Design review of the part built by this model. Coordinates are the model's own, in mm. A direction names the side the tool comes from. Round coordinates to 2 decimals unless told otherwise and drop trailing zeros. Loops run counter-clockwise (first coordinate to the right, second up) from the corner with the lowest first, then second, coordinate; pieces in that order, holes last. Notation, with made-up numbers: (33.5, -40) - (38.5, -40) arc R17 cw to (38.5, -20) - close; hole circle Ø7 at (65, 23.5). An arc over 180 degrees is marked (long way). Return JSON: item names as keys, results as strings. Group by question number.
(1) Wall thickness on L1, parallel to X at y = 4.75, z = 0; L2, parallel to X at y = -10, z = 11.5; L3, parallel to Y at x = 57, z = -0.5: over which ranges is each line inside the solid? List them lowest first. Write a range as [from, to].
(2) For faces 1 (the flat face through (68.58, 0, 0)), 2 (the cylindrical face through (36.403, -7.559, -5.796)), list the 3-axis set-ups (+Z, -Z, +X, -X, +Y, -Y) from which the entire face can be reached by the end or side of a thin tool; tool diameter is ignored.
(3) We need section C-C, the plane x = 24. Write out the cut boundary in (y, z) (3 decimals), and give its area (3 significant figures).
(4) Clearance check with flat-ended pins moving along their axes: pin 1 (10 mm diameter, centred on x = 60.5, z = -10.5, fed in from +Y); pin 2 (8 mm diameter, centred on x = 55, z = 5.5, fed in from -Y); pin 3 (3 mm diameter, centred on x = 16, z = 5, fed in from +Y); pin 4 (4.5 mm diameter, centred on x = 59.95, z = 0, fed in from -Y). State where each tip first meets the part, or that it passes through.
(5) We need section D-D, the plane z = -11.5. Write out the cut boundary in (x, y).
(6) We need section A-A, the plane z = 0. Write out the cut boundary in (x, y) (3 decimals).
(7) The part is to be moulded in two halves that separate along X. For faces 3 (the cylindrical face through (57.566, -0.133, 0.105)), 4 (the flat face through (6.35, 7, -7)), 5 (the cylindrical face through (3.131, -3.441, -15.497)), say which applies: pulls with the +X half, pulls with the -X half, needs draft (parallel to the pull), parting line crosses it, or undercut.
(8) We need section B-B, the plane y = 0. Write out the cut boundary in (x, z) (3 decimals).
from build123d import *

# Parameters (mm, degrees)
F0_R     = 15.875
F1_DEPTH = 6.35
F2_R     = 9.525
F3_DEPTH = 62.23
F4_R     = 1.27
F5_R     = 2.3876
F6_DEPTH = 12.7


with BuildPart() as f1:
    # F0 (on Right) → F1 (new body)
    with BuildSketch(Plane.YZ):
        Circle(F0_R)
    extrude(amount=F1_DEPTH)

    # F2 (on face) → F3 (join)
    with BuildSketch(Plane.YZ.offset(6.35)):
        Circle(F2_R)
    extrude(amount=F3_DEPTH)

    # F4
    f4_edges = [f1.edges().sort_by_distance(p)[0] for p in [
        (68.58, -9.525, 0),
    ]]
    fillet(f4_edges, radius=F4_R)

    # F5 (on Front) → F6 (cut, symmetric)
    with BuildSketch(Plane.XZ):
        with Locations((59.951451, 0)):
            Circle(F5_R)
    extrude(amount=F6_DEPTH, both=True, mode=Mode.SUBTRACT)


solid = f1.part
Solutions:
{
 "1": {"L1": "[0, 57.56], [62.34, 68.58]", "L2": "[0, 6.35]", "L3": "[-9.51, 9.51]"},
 "2": {"face 1": "+Z, -Z, +X, +Y, -Y", "face 2": "+X"},
 "3": {"outline": "circle Ø19.05 at (0, 0)", "area": "285 mm^2"},
 "4": {"pin 1": "y = 7.78", "pin 2": "y = -9.41", "pin 3": "y = 8.86", "pin 4": "through"},
 "5": {"outline": "(0, -10.94) - (6.35, -10.94) - (6.35, 10.94) - (0, 10.94) - close"},
 "6": {"outline": "(0, -15.875) - (6.35, -15.875) - (6.35, -9.525) - (57.564, -9.525) - (57.564, 9.525) - (6.35, 9.525) - (6.35, 15.875) - (0, 15.875) - close; (62.339, -9.525) - (67.31, -9.525) arc R1.27 ccw to (68.58, -8.255) - (68.58, 8.255) arc R1.27 ccw to (67.31, 9.525) - (62.339, 9.525) - close"},
 "7": {"face 3": "undercut", "face 4": "pulls with the +X half", "face 5": "needs draft"},
 "8": {"outline": "(0, -15.875) - (6.35, -15.875) - (6.35, -9.525) - (67.31, -9.525) arc R1.27 ccw to (68.58, -8.255) - (68.58, 8.255) arc R1.27 ccw to (67.31, 9.525) - (6.35, 9.525) - (6.35, 15.875) - (0, 15.875) - close; hole circle Ø4.775 at (59.951, 0)"}
}
